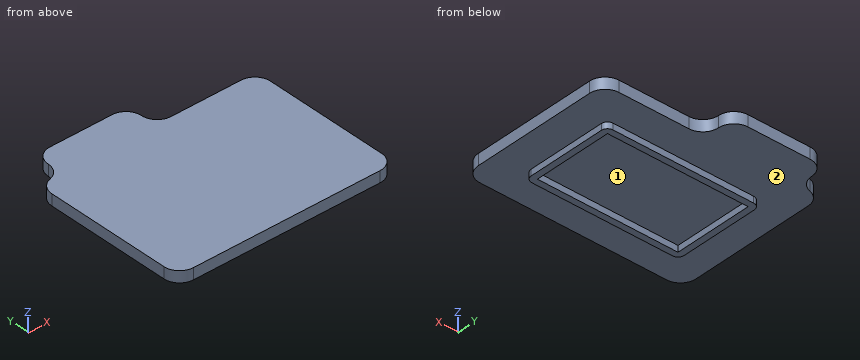
Autodesk Inventor part; units mm, degrees
ref_plane "YZ Plane" through (0, 0, 0) normal (1, 0, 0) x (0, 1, 0)
ref_plane "XZ Plane" through (0, 0, 0) normal (0, 1, 0) x (-1, 0, 0)
ref_plane "XY Plane" through (0, 0, 0) normal (0, 0, 1) x (1, 0, 0)
sketch "Sketch4" plane through (0, 0, 0) normal (0, 0, 1) x (1, 0, 0)
  line L0 (15.875, 9.525) -> (15.875, -9.525)
  line L1 (15.875, -9.525) -> (-15.875, -9.525)
  line L2 (-15.875, -9.525) -> (-15.875, 9.525)
  line L3 (-15.875, 9.525) -> (-11.1125, 9.525)
  line L4 (-11.1125, 9.525) -> (-11.1125, 15.875)
  line L5 (-11.1125, 15.875) -> (-4.7625, 15.875)
  line L6 (-4.7625, 15.875) -> (-4.7625, 9.525)
  line L7 (-4.7625, 9.525) -> (15.875, 9.525)
  line L8 (1.5875, 22.225) -> (-17.4625, 22.225)
  line L9 (-17.4625, 22.225) -> (-17.4625, 15.875)
  line L10 (-17.4625, 15.875) -> (-22.225, 15.875)
  line L11 (-22.225, 15.875) -> (-22.225, -15.875)
  line L12 (-22.225, -15.875) -> (22.225, -15.875)
  line L13 (22.225, -15.875) -> (22.225, 15.875)
  line L14 (22.225, 15.875) -> (1.5875, 15.875)
  line L15 (1.5875, 15.875) -> (1.5875, 22.225)
  circle A0 centre (-14.2875, 19.05) radius 1.7145
  circle A1 centre (-1.5875, 19.05) radius 1.7145
  circle A2 centre (-1.5875, 12.7) radius 1.7145
  circle A3 centre (7.9375, 12.7) radius 1.7145
  circle A4 centre (19.05, 12.7) radius 1.7145
  circle A5 centre (19.05, 0) radius 1.7145
  circle A6 centre (19.05, -12.7) radius 1.7145
  circle A7 centre (-19.05, 0) radius 1.7145
  circle A8 centre (-19.05, -12.7) radius 1.7145
  circle A9 centre (-9.525, -12.7) radius 1.7145
  circle A10 centre (0, -12.7) radius 1.7145
  circle A11 centre (9.525, -12.7) radius 1.7145
  circle A12 centre (-19.05, 12.7) radius 1.7145
  point P0 (0, 0)
  dimension "d95" = 3.429
  dimension "d96" = 3.429
  dimension "d97" = 3.429
  dimension "d98" = 3.429
  dimension "d99" = 3.429
  dimension "d100" = 3.429
  dimension "d101" = 3.429
  dimension "d102" = 3.429
  dimension "d103" = 3.429
  dimension "d104" = 3.429
  dimension "d105" = 3.429
  dimension "d106" = 3.429
  dimension "d107" = 3.175
  dimension "d108" = 3.175
  dimension "d109" = 3.175
  dimension "d110" = 3.175
  dimension "d111" = 3.175
  dimension "d112" = 3.175
  dimension "d113" = 9.525
  dimension "d114" = 9.525
  dimension "d115" = 9.525
  dimension "d116" = 9.525
  dimension "d117" = 3.429
  dimension "d118" = 3.175
  dimension "d119" = 3.175
extrude "Extrusion4" add sketch "Sketch4" along normal blind 2.286 contours L0 L1 L2 L3 L4 L5 L6 L7 | L15 L14 L13 L12 L11 L10 L9 L8 | A0 | A1 | A2 | A3 | A4 | A5 | A6 | A7 | A8 | A9 | A10 | A11 | A12
fillet "Fillet3" radius 3.175 8 edges at (-17.4625, 22.225, 1.143) (1.5875, 22.225, 1.143) (1.5875, 15.875, 1.143) (-17.4625, 15.875, 1.143) (-22.225, 15.875, 1.143) (22.225, 15.875, 1.143) (22.225, -15.875, 1.143) (-22.225, -15.875, 1.143)
sketch "Sketch5" plane through (0, 0, 0) normal (0, 0, -1) x (-1, 0, 0)
  arc A0 (19.05, -15.875) -> (22.225, -12.7) centre (19.05, -12.7) ccw construction
  line L0 (22.225, -12.7) -> (22.225, 12.9016) construction
  arc A1 (22.225, 12.9016) -> (19.8438, 15.9758) centre (19.05, 12.9016) ccw construction
  arc A2 (17.4625, 19.05) -> (19.8438, 15.9758) centre (20.6375, 19.05) ccw construction
  arc A3 (17.4625, 19.05) -> (14.2875, 22.225) centre (14.2875, 19.05) ccw construction
  line L1 (14.2875, 22.225) -> (1.5875, 22.225) construction
  arc A4 (1.5875, 22.225) -> (-1.5875, 19.05) centre (1.5875, 19.05) ccw construction
  arc A5 (-4.7625, 15.875) -> (-1.5875, 19.05) centre (-4.7625, 19.05) ccw construction
  line L2 (-4.7625, 15.875) -> (-19.05, 15.875) construction
  arc A6 (-19.05, 15.875) -> (-22.225, 12.7) centre (-19.05, 12.7) ccw construction
  line L3 (-22.225, 12.7) -> (-22.225, -12.7) construction
  arc A7 (-22.225, -12.7) -> (-19.05, -15.875) centre (-19.05, -12.7) ccw construction
  line L4 (-19.05, -15.875) -> (19.05, -15.875) construction
  line L5 (-15.621, 9.271) -> (15.621, 9.271)
  line L6 (15.621, 9.271) -> (15.621, -9.271)
  line L7 (15.621, -9.271) -> (-15.621, -9.271)
  line L8 (-15.621, -9.271) -> (-15.621, 9.271)
  line L9 (14.351, 8.001) -> (-14.351, 8.001)
  line L10 (-14.351, 8.001) -> (-14.351, -8.001)
  line L11 (-14.351, -8.001) -> (14.351, -8.001)
  line L12 (14.351, -8.001) -> (14.351, 8.001)
  point P0 (0, 0)
  dimension "d126" = 6.604
  dimension "d127" = 6.604
  dimension "d128" = 6.604
  dimension "d129" = 6.604
  dimension "d130" = 1.27
extrude "Extrusion5" add sketch "Sketch5" along normal blind 1.27
fillet "Fillet4" radius 1.27 4 edges at (-15.621, 9.271, -0.635) (-15.621, -9.271, -0.635) (15.621, -9.271, -0.635) (15.621, 9.271, -0.635)
equation "\"d95\" = d117"
equation "\"d96\" = d117"
equation "\"d97\" = d117"
equation "\"d98\" = d117"
equation "\"d99\" = d117"
equation "\"d100\" = d117"
equation "\"d101\" = d117"
equation "\"d102\" = d117"
equation "\"d103\" = d117"
equation "\"d104\" = d117"
equation "\"d105\" = d117"
equation "\"d106\" = d117"
equation "\"d115\" = d114"
equation "\"d116\" = d114"
properties part number "foreElectronicsSealingWallFrontCap" material "ABS Plastic"
Build history of the part. All positions in model axes, mm. Face numbers are marked on the shaded views. Coordinates: 2 decimals unless noted, no trailing zeros. Order: outer loops, then holes, each group sorted by start corner. A loop starts at its lowest first (then second) coordinate and runs counter-clockwise, first axis right, second up. Notation, with made-up numbers: (-34, 86) - (0, 86) arc R11 ccw to (0, 103) - close; hole circle Ø11 at (-0.5, -31.5). An arc over 180 degrees is marked (long way). Put each result on its own line as item: value.
1. Pull direction Y, two halves, no side cores. Call the marked faces 1 and 2: pulls with the +Y half, pulls with the -Y half, needs draft (parallel to the pull), parting line crosses it, or undercut.
Answer sheet:
face 1: undercut
face 2: needs draft
2. Saw through at A-A (z = -0.8). Write the cut outline in (x, y), and give its area (3 significant figures).
Answer sheet:
outline: (-15.62, -8) arc R1.27 ccw to (-14.35, -9.27) - (14.35, -9.27) arc R1.27 ccw to (15.62, -8) - (15.62, 8) arc R1.27 ccw to (14.35, 9.27) - (-14.35, 9.27) arc R1.27 ccw to (-15.62, 8) - close; hole (-14.35, -8) - (14.35, -8) - (14.35, 8) - (-14.35, 8) - close
area: 119 mm^2
3. Drop flat-ended pins along their axis: P1, Ø0.6, axis at x = -7, z = -1, coming from the +Y side; P2, Ø8, axis at x = 5, y = -2.5, coming from the -Z side; P3, Ø0.6, axis at y = -2, z = -1, coming from the +X side. Give the stop position or say it passes through.
Answer sheet:
P1: stops at y = 9.27
P2: stops at z = 0
P3: stops at x = 15.62
4. Probe line 1 along Y through (x, z) = (-1.5, -1); line 2 along X through (y, z) = (-1.5, -0.1); line 3 along Z through (x, y) = (-5.5, -3). List the from-to ranges inside material, lowest first. Write a range as [from, to].
Answer sheet:
line 1: y = [-9.27, -8], [8, 9.27]
line 2: x = [-15.62, -14.35], [14.35, 15.62]
line 3: z = [0, 2.29]
5. Saw through at B-B (x = 6.5). Write the cut outline in (y, z) (3 decimals).
Answer sheet:
outline: (-15.875, 0) - (-9.271, 0) - (-9.271, -1.27) - (-8.001, -1.27) - (-8.001, 0) - (8.001, 0) - (8.001, -1.27) - (9.271, -1.27) - (9.271, 0) - (15.875, 0) - (15.875, 2.286) - (-15.875, 2.286) - close
6. Saw through at D-D (y = -8.5). Write the cut outline in (x, z) (3 decimals).
Answer sheet:
outline: (-22.225, 0) - (-15.519, 0) - (-15.519, -1.27) - (15.519, -1.27) - (15.519, 0) - (22.225, 0) - (22.225, 2.286) - (-22.225, 2.286) - close
7. Saw through at C-C (y = 7). Write the cut outline in (x, z) (3 decimals), and give its area (3 significant figures).
Answer sheet:
outline: (-22.225, 0) - (-15.621, 0) - (-15.621, -1.27) - (-14.351, -1.27) - (-14.351, 0) - (14.351, 0) - (14.351, -1.27) - (15.621, -1.27) - (15.621, 0) - (22.225, 0) - (22.225, 2.286) - (-22.225, 2.286) - close
area: 105 mm^2
